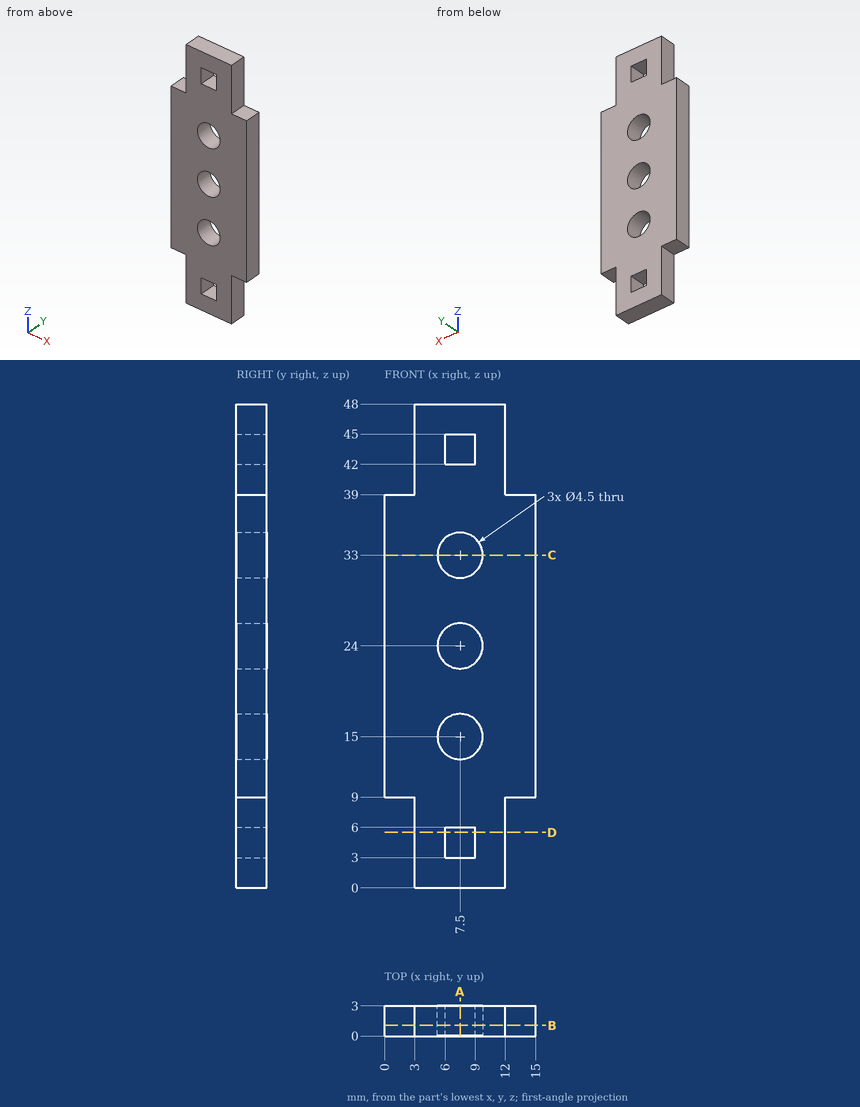
Geometry: see drawing. Coordinates: mm, zero at the bounding-box minimum. Round coordinates to 2 decimals unless told otherwise and drop trailing zeros. Loops run counter-clockwise (first coordinate to the right, second up) from the corner with the lowest first, then second, coordinate; pieces in that order, holes last. Notation, with made-up numbers: M 80,53.5 L 137,53.5 A18 ccw 137,88.5 Z; hole C 68,24 d10. An arc over 180 degrees is marked long. Use a Markdown table: item, result. Add a question column.
1. Contact query for flat-ended pins moving along their axis: P1, Ø0.9, axis at y = 2, z = 45, coming from the +X side; P2, Ø1.5, axis at x = 14, y = 1.5, coming from the +Z side; P3, Ø1.5, axis at y = 1.5, z = 5, coming from the -X side. Output: stop coordinate, or through.
2. Line query: line 1 (Z direction, x = 7.5, y = 2.05); line 2 (X direction, y = 1.7, z = 44.5); line 3 (Z direction, x = 5.5, y = 1.95). Output: solid intervals per line, ascending.
3. Section query B-B on y = 1.05. Return the cut outline in (x, z).
4. Section query A-A on x = 7.5. Return the cut outline in (y, z), then the cut area to 3 significant figures.
5. Section query C-C on z = 33. Return the cut outline in (x, y).
6. Section query D-D on z = 5.5. Return the cut outline in (x, y), then the cut area to 3 significant figures.
Reported:
| question | item | result |
|---|---|---|
| 1 | P1 | stops at x = 12 |
| 1 | P2 | stops at z = 39 |
| 1 | P3 | stops at x = 3 |
| 2 | line 1 | z = 0 to 3, 6 to 12.75, 17.25 to 21.75, 26.25 to 30.75, 35.25 to 42, 45 to 48 |
| 2 | line 2 | x = 3 to 6, 9 to 12 |
| 2 | line 3 | z = 0 to 13.97, 16.03 to 22.97, 25.03 to 31.97, 34.03 to 48 |
| 3 | outline | M 0,9 L 3,9 L 3,0 L 12,0 L 12,9 L 15,9 L 15,39 L 12,39 L 12,48 L 3,48 L 3,39 L 0,39 Z; hole C 7.5,15 d4.5; hole C 7.5,24 d4.5; hole C 7.5,33 d4.5; hole M 6,3 L 9,3 L 9,6 L 6,6 Z; hole M 6,42 L 9,42 L 9,45 L 6,45 Z |
| 4 | outline | M 0,0 L 3,0 L 3,3 L 0,3 Z; M 0,6 L 3,6 L 3,12.75 L 0,12.75 Z; M 0,17.25 L 3,17.25 L 3,21.75 L 0,21.75 Z; M 0,26.25 L 3,26.25 L 3,30.75 L 0,30.75 Z; M 0,35.25 L 3,35.25 L 3,42 L 0,42 Z; M 0,45 L 3,45 L 3,48 L 0,48 Z |
| 4 | area | 85.5 mm² |
| 5 | outline | M 0,0 L 5.25,0 L 5.25,3 L 0,3 Z; M 9.75,0 L 15,0 L 15,3 L 9.75,3 Z |
| 6 | outline | M 3,0 L 6,0 L 6,3 L 3,3 Z; M 9,0 L 12,0 L 12,3 L 9,3 Z |
| 6 | area | 18.0 mm² |
